Could you check a few things on this drawing? It's one solid part, dimensions in mm from its lowest x, y, z. Coordinates: 2 decimals unless noted, no trailing zeros. Order: outer loops, then holes, each group sorted by start corner. A loop starts at its lowest first (then second) coordinate and runs counter-clockwise, first axis right, second up. Notation, with made-up numbers: (-33, 77) -> (-11, 77) arc R8 cw to (-11, 84) -> close; hole circle Ø5 at (67, 71). An arc over 180 degrees is marked (long way). Use a Markdown table: item, result. Add a question column.
1. For pin 1 Ø10 at (x, z) = (54, 93) entering from -Y; pin 2 Ø4 at (x, y) = (155, 34.5) entering from +Z; pin 3 Ø7.5 at (x, y) = (115, 290) entering from +Z, each with a flat end and sliding along its axis, tell me the tip position at first contact or that it passes through.
2. If I drill on line 1 along X through (y, z) = (225, 136.5); line 2 along Y through (x, z) = (38.5, 15); line 3 along Y through (x, z) = (280.5, 82), over which ranges is the centre line in solid material (lowest first)? Write a range as from..to.
3. We'd pull the mould along Y, two halves only. Please class the marked faces 1, 2 and 3: pulls with the +Y half, pulls with the -Y half, needs draft (parallel to the pull), parting line crosses it, or undercut.
4. Suppose I cut it at B-B, the plane y = 26.5. List the corners of the cut face in (x, z) for me, then the cut area to 3 significant figures.
5. Suppose I cut it at C-C, the plane x = 305. List the corners of the cut face in (y, z) for me.
6. Suppose I cut it at A-A, the plane z = 60. List the corners of the cut face in (x, y) for me.
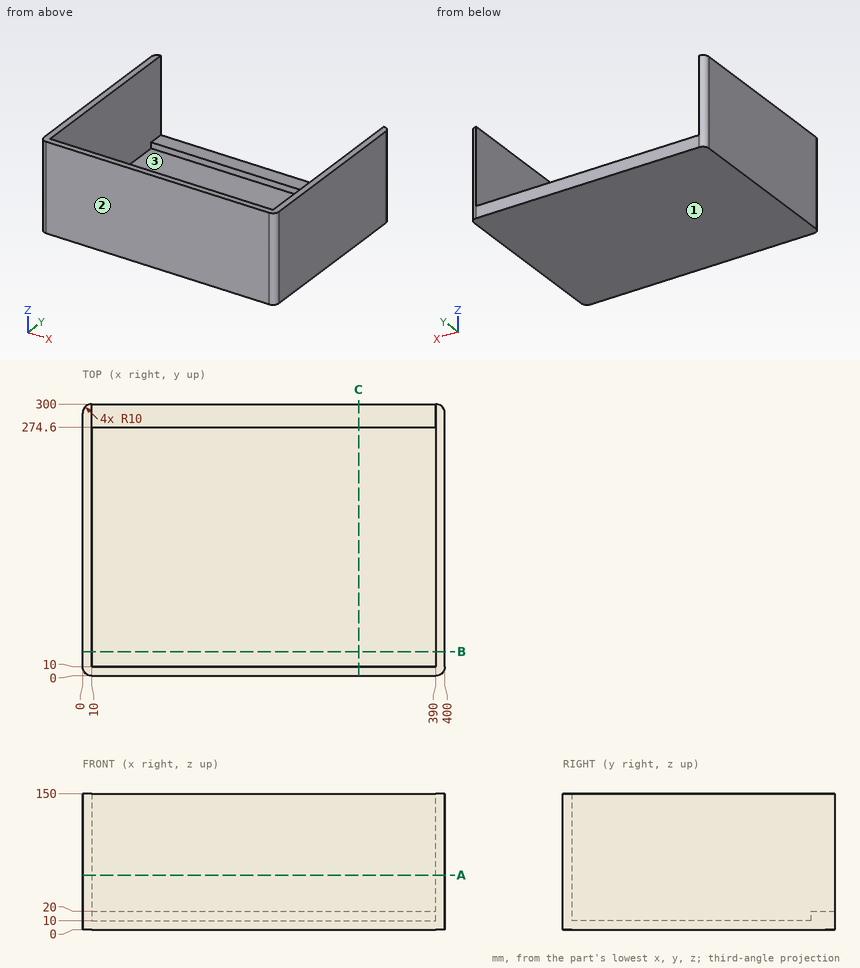
Worked out:
| question | item | result |
|---|---|---|
| 1 | pin 1 | stops at y = 0 |
| 1 | pin 2 | stops at z = 10 |
| 1 | pin 3 | stops at z = 20 |
| 2 | line 1 | x = 0..10, 390..400 |
| 2 | line 2 | y = 0..10, 274.6..300 |
| 2 | line 3 | y = 0..10 |
| 3 | face 1 | needs draft |
| 3 | face 2 | pulls with the -Y half |
| 3 | face 3 | undercut |
| 4 | outline | (0, 0) -> (400, 0) -> (400, 150) -> (390, 150) -> (390, 10) -> (10, 10) -> (10, 150) -> (0, 150) -> close |
| 4 | area | 6,800 mm² |
| 5 | outline | (0, 0) -> (300, 0) -> (300, 20) -> (274.6, 20) -> (274.6, 10) -> (10, 10) -> (10, 150) -> (0, 150) -> close |
| 6 | outline | (0, 10) arc R10 ccw to (10, 0) -> (390, 0) arc R10 ccw to (400, 10) -> (400, 290) arc R10 ccw to (390, 300) -> (390, 10) -> (10, 10) -> (10, 300) arc R10 ccw to (0, 290) -> close |
